The model under review builds one solid part; all positions refer to its coordinate system, in mm. A direction names the side the tool comes from. Coordinates: 2 decimals unless noted, no trailing zeros. Write each loop counter-clockwise with the first axis right and the second up, starting at its lowest first coordinate (ties: lowest second). Pieces come first, ordered by that corner, then holes. Notation, with made-up numbers: (33.25, 88) -> (76.25, 88) arc R34 ccw to (76.25, 127) -> close; hole circle Ø2 at (35, 50). An arc over 180 degrees is marked (long way). Write each question's results on one line, items separated by ' | '.
```python
from build123d import *

# Parameters (mm, degrees)
F0_W     = 304.8
F0_H     = 121.92
F1_DEPTH = 304.8
F2_W     = 236.021310091
F2_H     = 246.3743686676
F3_DEPTH = 73.152
F4_R     = 69.9059679121
F5_R     = 107.4455989459
F6_DEPTH = 79.248
F7_R     = 7.3585229381
F8_W     = 48.9512532949
F8_H     = 10.1278424263
F9_DEPTH = 10.668


with BuildPart() as f1:
    # F0 (on Top) → F1 (new body)
    with BuildSketch(Plane.XY):
        with Locations((152.4, -60.96)):
            Rectangle(F0_W, F0_H)
    extrude(amount=F1_DEPTH)

    # F2 (on Top) → F3 (join, symmetric)
    with BuildSketch(Plane.XY):
        with Locations((152.538523078, 123.1871843338)):
            Rectangle(F2_W, F2_H)
    extrude(amount=F3_DEPTH, both=True)

    # F4
    f4_edges = [f1.edges().sort_by_distance(p)[0] for p in [
        (34.527868, 246.374369, 0),
        (270.549178, 246.374369, 0),
        (34.527868, 0, -36.576),
        (270.549178, 0, -36.576),
    ]]
    fillet(f4_edges, radius=F4_R)

    # F5 (on face) → F6 (cut)
    with BuildSketch(Plane.XY.offset(73.152)):
        with Locations((152.538523078, 121.3710904121)):
            Circle(F5_R)
    extrude(amount=-F6_DEPTH, mode=Mode.SUBTRACT)

    # F7
    f7_edges = [f1.edges().sort_by_distance(p)[0] for p in [
        (304.8, -60.96, 304.8),
        (0, -60.96, 304.8),
    ]]
    fillet(f7_edges, radius=F7_R)

    # F8 (on face) → F9 (join)
    with BuildSketch(Plane(origin=(0, 0, 0), x_dir=(-1, 0, 0), z_dir=(0, 1, 0))):
        with Locations((-264.9517431855, 283.5146784782)):
            Rectangle(F8_W, F8_H)
    extrude(amount=F9_DEPTH)


solid = f1.part
```
Q1. Machinability: for faces 1 (the flat face through (265, 10.668, 284)), 2 (the flat face through (34.528, 107, 17)), 3 (the flat face through (240.476, 5, 283)), 4 (the flat face through (151, 123, -6.096)), 5 (the cylindrical face through (54.462, 21.021, -36.064)), which of the approach directions +Z, -Z, +X, -X, +Y, -Y give a long, thin tool a straight path to every point of the face, cutting with its end or side? Answer none if there is none.
Solution:
face 1: +Z, +X, -X, +Y | face 2: +Z, -Z, -X, +Y | face 3: +Z, -X, +Y | face 4: +Z | face 5: -Z, -X, -Y
Q2. Add section B-B (z = -40). Write out the cut boundary in (x, y).
Solution:
outline: (34.53, 69.91) arc R69.91 ccw to (104.43, 0) -> (200.64, 0) arc R69.91 ccw to (270.55, 69.91) -> (270.55, 176.47) arc R69.91 ccw to (200.64, 246.37) -> (104.43, 246.37) arc R69.91 ccw to (34.53, 176.47) -> close
Q3. For line 1 (Y direction, x = 149, z = 27); line 2 (Z direction, x = 102, y = 64); line 3 (Z direction, x = 255, y = 68), list the stretches that pass through material, from the lowest coordinate up. Write a range as from..to.
Solution:
line 1: -121.92..13.98, 228.76..246.37 | line 2: -73.15..-6.1 | line 3: -73.15..73.15
Q4. Draft analysis for pull direction Z (two halves, no side actions). For faces 6 (the flat face through (265, 5, 278.451)), 7 (the flat face through (0, -62, 147)), 8 (the flat face through (265, 5, 288.579)), state which applies: pulls with the +Z half, pulls with the -Z half, needs draft (parallel to the pull), parting line crosses it, or undercut.
Solution:
face 6: undercut | face 7: needs draft | face 8: pulls with the +Z half
Q5. Clearance check with flat-ended pins moving along their axes: P1, Ø11, axis at y = 7, z = 281.5, coming from the +X side; P2, Ø3, axis at x = 265.5, y = 7.5, coming from the -Z side; P3, Ø3, axis at y = 5.5, z = 285.5, coming from the -X side. State where each tip first meets the part, or that it passes through.
Solution:
P1: x = 289.43 | P2: z = 0 | P3: x = 240.48
Q6. Add section A-A (x = 278.5). Write out the cut boundary in (y, z), plus the area to 3 significant figures.
Solution:
outline: (-121.92, 0) -> (0, 0) -> (0, 278.45) -> (10.67, 278.45) -> (10.67, 288.58) -> (0, 288.58) -> (0, 304.8) -> (-121.92, 304.8) -> close | area: 37,300 mm²
Q7. Add section D-D (z = 41). Write out the cut boundary in (x, y), plus the area to 3 significant figures.
Solution:
outline: (0, -121.92) -> (304.8, -121.92) -> (304.8, 0) -> (270.55, 0) -> (270.55, 176.47) arc R69.91 ccw to (200.64, 246.37) -> (104.43, 246.37) arc R69.91 ccw to (34.53, 176.47) -> (34.53, 0) -> (0, 0) -> close; hole circle Ø214.89 at (152.54, 121.37) | area: 56,900 mm²
Q8. Add section C-C (y = 64.5). Write out the cut boundary in (x, z), plus the area to 3 significant figures.
Solution:
outline: (34.53, 0) -> (34.74, 0) -> (34.74, -73.15) -> (270.34, -73.15) -> (270.34, 0) -> (270.55, 0) -> (270.55, 73.15) -> (243.7, 73.15) -> (243.7, -6.1) -> (61.38, -6.1) -> (61.38, 73.15) -> (34.53, 73.15) -> close | area: 20,100 mm²
